Drawing for the job (mm, zero at the part's lowest x, y, z). A direction names the side the tool comes from. Round coordinates to 2 decimals unless told otherwise and drop trailing zeros. Order: outer loops, then holes, each group sorted by start corner. A loop starts at its lowest first (then second) coordinate and runs counter-clockwise, first axis right, second up. Notation, with made-up numbers: (-37.5, -20.5) -> (-3.5, -20.5) arc R28 cw to (-3.5, 7.5) -> close; hole circle Ø2 at (73, 84). An arc over 180 degrees is marked (long way). Use CSV: the item, a comma, the result in double quotes.
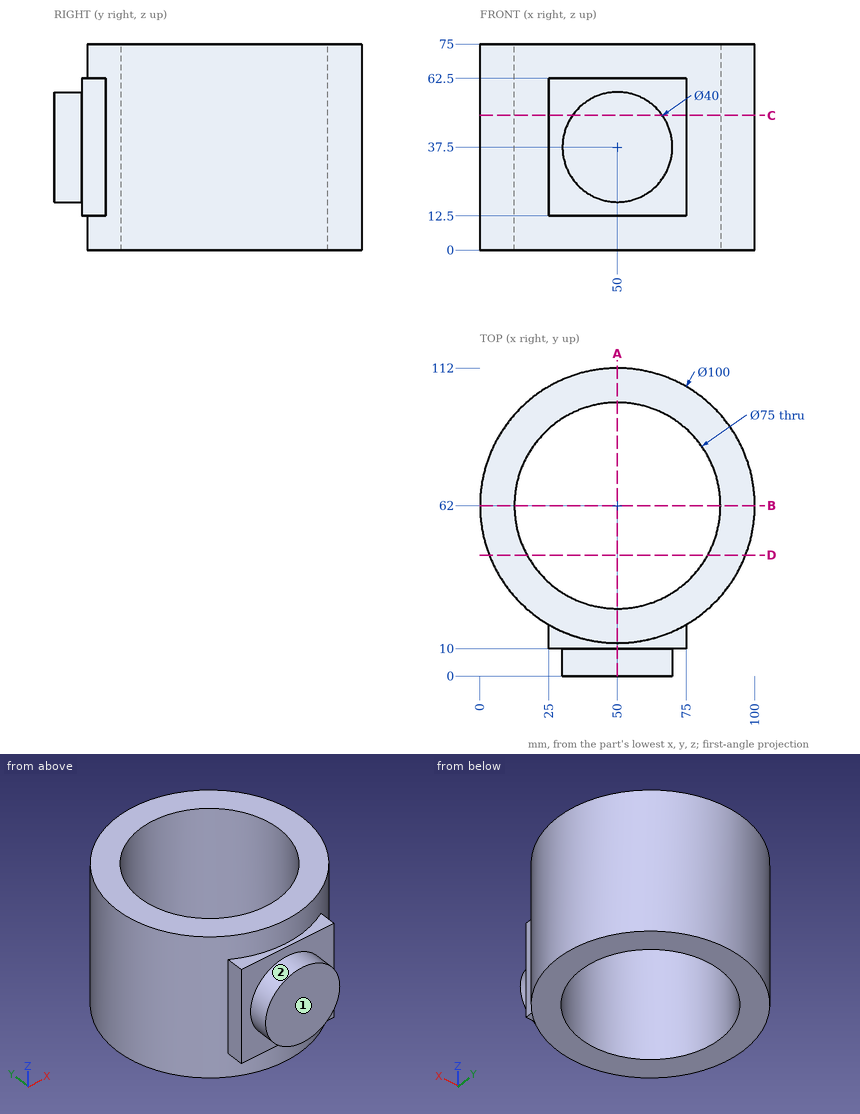
Q1. Cut at A-A (x = 50). Give the cut face in (y, z).
From the geometry:
outline,"(0, 17.5) -> (10, 17.5) -> (10, 12.5) -> (12, 12.5) -> (12, 0) -> (24.5, 0) -> (24.5, 75) -> (12, 75) -> (12, 62.5) -> (10, 62.5) -> (10, 57.5) -> (0, 57.5) -> close; (99.5, 0) -> (112, 0) -> (112, 75) -> (99.5, 75) -> close"
Q2. Cut at B-B (y = 62). Give the cut face in (x, z).
From the geometry:
outline,"(0, 0) -> (12.5, 0) -> (12.5, 75) -> (0, 75) -> close; (87.5, 0) -> (100, 0) -> (100, 75) -> (87.5, 75) -> close"
Q3. Cut at C-C (z = 49). Give the cut face in (x, y).
From the geometry:
outline,"(25, 10) -> (33.64, 10) -> (33.64, 0) -> (66.36, 0) -> (66.36, 10) -> (75, 10) -> (75, 18.7) arc R50 ccw (long way) to (25, 18.7) -> close; hole circle Ø75 at (50, 62)"
Q4. Probe line 1 along Y through (x, z) = (50, 49); line 2 along X through (y, z) = (34.5, 60); line 3 along Y through (x, z) = (81, 59). List the from-to ranges inside material, lowest first.
From the geometry:
line 1,"y = 0 to 24.5, 99.5 to 112"
line 2,"x = 8.24 to 24.5, 75.5 to 91.76"
line 3,"y = 22.77 to 40.9, 83.1 to 101.23"
Q5. Pin check, flat tips, straight feed: pin 1 (7 mm diameter, centred on y = 14.5, z = 37.5, fed in from +X); pin 2 (12 mm diameter, centred on y = 72, z = 42.5, fed in from -X); pin 3 (2 mm diameter, centred on y = 81, z = 23.5, fed in from +X). Stop position of each tip, or through.
From the geometry:
pin 1,"stops at x = 75"
pin 2,"stops at x = 0.16"
pin 3,"stops at x = 96.65"
Q6. Cut at D-D (y = 44). Give the cut face in (x, z), plus the area to 3 significant figures.
From the geometry:
outline,"(3.35, 0) -> (17.1, 0) -> (17.1, 75) -> (3.35, 75) -> close; (82.9, 0) -> (96.65, 0) -> (96.65, 75) -> (82.9, 75) -> close"
area,"2,060 mm²"
Q7. Which spindle directions (+Z, -Z, +X, -X, +Y, -Y) get a long thin tool onto all of the face, cutting with end or side? Do the marked faces 1 and 2. Say none if no direction does.
From the geometry:
face 1,"+Z, -Z, +X, -X, -Y"
face 2,"-Y"
